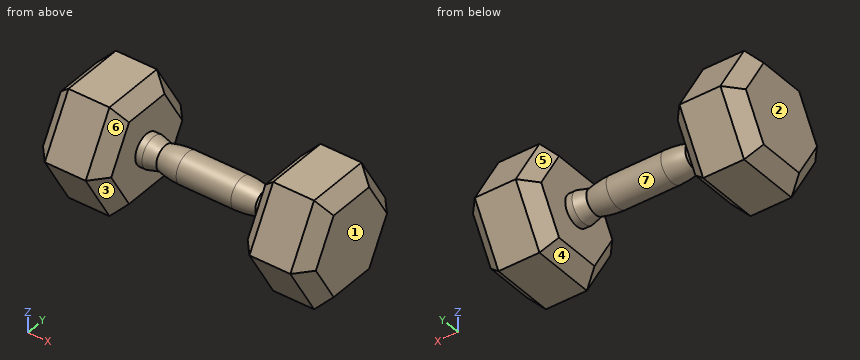
```python
from build123d import *

# Parameters (mm, degrees)
BOSS_EXTRUDE1_DEPTH = 63.5
CHAMFER1_SIZE       = 12.7
CHAMFER2_SIZE       = 12.7


with BuildPart() as part:
    # Sketch1 → Boss-Extrude1 (new body)
    with BuildSketch(Plane.YZ):
        Polygon((58.65878735, 0), (29.329393675, 50.8), (-29.329393675, 50.8), (-58.65878735, 0), (-29.329393675, -50.8), (29.329393675, -50.8), align=None)
    extrude(amount=BOSS_EXTRUDE1_DEPTH)

    # Chamfer1
    chamfer1_edges = [part.edges().sort_by_distance(p)[0] for p in [
        (63.5, 0, 50.8),
        (63.5, -43.994090512, 25.4),
        (63.5, -43.994090512, -25.4),
        (63.5, 0, -50.8),
        (63.5, 43.994090512, -25.4),
        (63.5, 43.994090512, 25.4),
    ]]
    chamfer(chamfer1_edges, length=CHAMFER1_SIZE)

    # Chamfer2
    chamfer2_edges = [part.edges().sort_by_distance(p)[0] for p in [
        (0, 0, -50.8),
        (0, -43.994090512, -25.4),
        (0, -43.994090512, 25.4),
        (0, 0, 50.8),
        (0, 43.994090512, 25.4),
        (0, 43.994090512, -25.4),
    ]]
    chamfer(chamfer2_edges, length=CHAMFER2_SIZE)

    # Sketch2 → Revolve1 (revolve)
    with BuildSketch(Plane(origin=(0, 0, 0), x_dir=(-1, 0, 0), z_dir=(0, 1, 0))):
        with BuildLine():
            Line((0, 0), (0, 14.2875))
            Line((0, 14.2875), (6.35, 14.2875))
            Line((6.35, 14.2875), (17.42833597, 11.43))
            ThreePointArc((17.42833597, 11.43), (27.66588528, 13.569744601), (38.1, 14.2875))
            Line((38.1, 14.2875), (63.5, 14.2875))
            Line((63.5, 14.2875), (63.5, 0))
            Line((63.5, 0), (0, 0))
        make_face()
    revolve(axis=Axis((-63.5, 0, 0), (1, 0, 0)))

    # Mirror1: part across plane


with BuildPart() as part_1:
    add(part.part)
    add(part.part.mirror(Plane(origin=(-63.5, 0, 14.2875), x_dir=(0, 0, 1), z_dir=(-1, 0, 0))))


solid = part_1.part
```
The model under review builds one solid part; all positions refer to its coordinate system, in mm. Face numbers are marked on the shaded views. A direction names the side the tool comes from. Round coordinates to 2 decimals unless told otherwise and drop trailing zeros. Order: outer loops, then holes, each group sorted by start corner. A loop starts at its lowest first (then second) coordinate and runs counter-clockwise, first axis right, second up. Notation, with made-up numbers: (29.25, -27.75) -> (40.25, -27.75) arc R19 ccw to (40.25, -19.75) -> close; hole circle Ø1 at (-34.5, 18). An arc over 180 degrees is marked (long way). Use a Markdown table: item, result.
Q1. We need section B-B on z = -18.5. Write out the cut boundary in (x, y), then the cut area to 3 significant figures.
Values:
| item | result |
|---|---|
| outline | (-190.5, -33.31) -> (-177.8, -47.98) -> (-139.7, -47.98) -> (-127, -33.31) -> (-127, 33.31) -> (-139.7, 47.98) -> (-177.8, 47.98) -> (-190.5, 33.31) -> close; (0, -33.31) -> (12.7, -47.98) -> (50.8, -47.98) -> (63.5, -33.31) -> (63.5, 33.31) -> (50.8, 47.98) -> (12.7, 47.98) -> (0, 33.31) -> close |
| area | 11,400 mm^2 |
Q2. For line 1 (X direction, y = 8.5, z = -12.5); line 2 (X direction, y = 40.5, z = -17); line 3 (Z direction, x = 28, y = 44), list the stretches that pass through material, from the lowest coordinate up.
Values:
| item | result |
|---|---|
| line 1 | x = -190.5 to -127, 0 to 63.5 |
| line 2 | x = -185.03 to -132.47, 5.47 to 58.03 |
| line 3 | z = -25.39 to 25.39 |
Q3. We need section A-A on y = -17.5. Write out the cut boundary in (x, z), then the cut area to 3 significant figures.
Values:
| item | result |
|---|---|
| outline | (-190.5, -38.1) -> (-177.8, -50.8) -> (-139.7, -50.8) -> (-127, -38.1) -> (-127, 38.1) -> (-139.7, 50.8) -> (-177.8, 50.8) -> (-190.5, 38.1) -> close; (0, -38.1) -> (12.7, -50.8) -> (50.8, -50.8) -> (63.5, -38.1) -> (63.5, 38.1) -> (50.8, 50.8) -> (12.7, 50.8) -> (0, 38.1) -> close |
| area | 12,300 mm^2 |
Q4. Mouldability with a two-part tool opening along X and no side actions: class the marked faces 1, 2 and 3 as +X half, -X half, draft (parallel to the pull), parting line (faces both ways), or undercut.
Values:
| item | result |
|---|---|
| face 1 | +X half |
| face 2 | -X half |
| face 3 | undercut |
Q5. Tool access review of the marked faces 4, 5, 6 and 7: name each direction out of +Z, -Z, +X, -X, +Y, -Y from which nothing blocks a thin tool from reaching the whole face with its end or side.
Values:
| item | result |
|---|---|
| face 4 | -Z, +Y, -Y |
| face 5 | +Z, +Y |
| face 6 | +Z, -Y |
| face 7 | none |
Q6. We need section D-D on y = 46.5. Write out the cut boundary in (x, z), then the cut area to 3 significant figures.
Values:
| item | result |
|---|---|
| outline | (-188.33, 0) -> (-177.8, -21.06) -> (-139.7, -21.06) -> (-129.17, 0) -> (-139.7, 21.06) -> (-177.8, 21.06) -> close; (2.17, 0) -> (12.7, -21.06) -> (50.8, -21.06) -> (61.33, 0) -> (50.8, 21.06) -> (12.7, 21.06) -> close |
| area | 4,100 mm^2 |
Q7. Clearance check with flat-ended pins moving along their axes: P1, Ø10, axis at y = 44.5, z = -24.5, coming from the -X side; P2, Ø8, axis at x = 23, z = -18.5, coming from the +Y side; P3, Ø3, axis at x = -5, z = -3, coming from the -Y side. State where each tip first meets the part, or that it passes through.
Values:
| item | result |
|---|---|
| P1 | stops at x = -182.81 |
| P2 | stops at y = 50.29 |
| P3 | stops at y = -14.21 |
Q8. We need section C-C on x = 29. Write out the cut boundary in (y, z).
Values:
| item | result |
|---|---|
| outline | (-58.66, 0) -> (-29.33, -50.8) -> (29.33, -50.8) -> (58.66, 0) -> (29.33, 50.8) -> (-29.33, 50.8) -> close |
